The listing builds one solid part. Answer for the finished solid, in the listing's coordinates (mm). A direction names the side the tool comes from. Round coordinates to 2 decimals unless told otherwise and drop trailing zeros. Loops run counter-clockwise (first coordinate to the right, second up) from the corner with the lowest first, then second, coordinate; pieces in that order, holes last. Notation, with made-up numbers: (44.5, 79) - (101.5, 79) arc R8 ccw to (101.5, 91) - close; hole circle Ø6 at (80, 72.5). An arc over 180 degrees is marked (long way). One line per item, written item: value.
```python
from build123d import *

# Parameters (mm, degrees)
SKETCH1_R           = 0.625
SKETCH1_R_2         = 1.875
BOSS_EXTRUDE1_DEPTH = 4
SKETCH2_R           = 4
CUT_EXTRUDE1_DEPTH  = 1.5


with BuildPart() as part:
    # Sketch1 → Boss-Extrude1 (new body)
    with BuildSketch(Plane(origin=(0, 0, 0), x_dir=(1, 0, 0), z_dir=(0, 1, 0))):
        with BuildLine():
            Line((-6, -4.5), (-11, -4.5))
            Line((-11, -4.5), (-11, -7.5))
            Line((-11, -7.5), (11, -7.5))
            Line((11, -7.5), (11, -4.5))
            Line((11, -4.5), (6, -4.5))
            ThreePointArc((6, -4.5), (0, 7.5), (-6, -4.5))
        make_face()
        with Locations((-7.05, -6)):
            Circle(SKETCH1_R, mode=Mode.SUBTRACT)
        with Locations((7.05, -6)):
            Circle(SKETCH1_R, mode=Mode.SUBTRACT)
        Circle(SKETCH1_R_2, mode=Mode.SUBTRACT)
    extrude(amount=BOSS_EXTRUDE1_DEPTH)

    # Sketch2 → Cut-Extrude1 (cut)
    with BuildSketch(Plane(origin=(0, 4, 0), x_dir=(1, 0, 0), z_dir=(0, 1, 0))):
        Circle(SKETCH2_R)
    extrude(amount=-CUT_EXTRUDE1_DEPTH, mode=Mode.SUBTRACT)


solid = part.part
```
1) For faces 4 (the cylindrical face through (-0.867, 3.26, 3.905)), 5 (the flat face through (9, 2, 4.5)), 6 (the flat face through (-8, 2, 4.5)), determine the directions among +Z, -Z, +X, -X, +Y, -Y from which every point of the face is accessible in a straight line to the end or side of a thin tool.
Final values:
face 4: +Y
face 5: +X, +Y, -Y
face 6: -X, +Y, -Y
2) A cutting plane is placed at A-A on z = 0. Give the vertices of the cut face in (x, y) (3 decimals).
Final values:
outline: (-7.5, 0) - (-1.875, 0) - (-1.875, 2.5) - (-4, 2.5) - (-4, 4) - (-7.5, 4) - close; (1.875, 0) - (7.5, 0) - (7.5, 4) - (4, 4) - (4, 2.5) - (1.875, 2.5) - close
3) A cutting plane is placed at D-D on x = -7.05. Give the vertices of the cut face in (y, z) (3 decimals), and give its area (3 significant figures).
Final values:
outline: (0, -2.559) - (4, -2.559) - (4, 2.559) - (0, 2.559) - close; (0, 4.5) - (4, 4.5) - (4, 5.375) - (0, 5.375) - close; (0, 6.625) - (4, 6.625) - (4, 7.5) - (0, 7.5) - close
area: 27.5 mm2
4) For a pull along X with two mould halves and no side action, classify faces 1 (the flat face through (0, 2, 7.5)), 2 (the flat face through (11, 2, 6)), 3 (the cylindrical face through (-1.873, 1.232, -0.082)) as released by +X, released by -X, zero draft, split by the parting line, or undercut.
Final values:
face 1: zero draft
face 2: released by +X
face 3: undercut
5) Each of these flat-tipped pins is pushed along its axis until it touches: pin 1 Ø2.5 at (x, z) = (-2, -1) entering from +Y; pin 2 Ø2 at (x, y) = (9, 3) entering from -Z; pin 3 Ø1.1 at (x, z) = (-7.05, 6) entering from -Y; pin 4 Ø2 at (x, y) = (-7.5, 1.5) entering from -Z. Where does it stop, or does it pass through?
Final values:
pin 1: y = 2.5
pin 2: z = 4.5
pin 3: through
pin 4: z = -3.74
6) A cutting plane is placed at C-C on x = 0. Give the vertices of the cut face in (y, z) (3 decimals), and give its area (3 significant figures).
Final values:
outline: (0, -7.5) - (4, -7.5) - (4, -4) - (2.5, -4) - (2.5, -1.875) - (0, -1.875) - close; (0, 1.875) - (2.5, 1.875) - (2.5, 4) - (4, 4) - (4, 7.5) - (0, 7.5) - close
area: 38.6 mm2
7) A cutting plane is placed at B-B on y = 0.75. Give the vertices of the cut face in (x, z) (3 decimals).
Final values:
outline: (-11, 4.5) - (-6, 4.5) arc R7.5 ccw (long way) to (6, 4.5) - (11, 4.5) - (11, 7.5) - (-11, 7.5) - close; hole circle Ø1.25 at (-7.05, 6); hole circle Ø3.75 at (0, 0); hole circle Ø1.25 at (7.05, 6)
8) Consider L1, parallel to X at y = 1.3, z = 0 (3 decimals); L2, parallel to X at y = 2.4, z = 6 (3 decimals); L3, parallel to X at y = 2.8, z = 0. Determine where each line is inside the solid, lowest interval first.
Final values:
L1: -7.5 to -1.875, 1.875 to 7.5
L2: -11 to -7.675, -6.425 to 6.425, 7.675 to 11
L3: -7.5 to -4, 4 to 7.5
